Here's how the part is built. I have some questions about the finished solid (model axes, mm). A direction names the side the tool comes from. Coordinates: 2 decimals unless noted, no trailing zeros. Write each loop counter-clockwise with the first axis right and the second up, starting at its lowest first coordinate (ties: lowest second). Pieces come first, ordered by that corner, then holes.
(1) Thinking about a two-plate mould opening in X: for faces 1 (the cylindrical face through (4.77, 1.23, 1.5)), 2 (the flat face through (6, 0.5, -0.5)), 3 (the cylindrical face through (6.677, 1.972, -2.103)), which applies, released by +X, released by -X, zero draft, split by the parting line, or undercut?
(2) Imagine slicing it at B-B, the plane x = 0. List the corners of the cut face in (y, z) for me.
(3) Please list where these lines run through material, in increasing order: probe 1 along Z at (x, y) = (0, 0.9); probe 2 along Y at (x, z) = (-1, 5); probe 3 along X at (y, z) = (1.4, 3).
(4) Which directions (+Z, -Z, +X, -X, +Y, -Y) give clear straight access to the entire face, cutting with the end or side of a thin tool? Please do faces 4 (the flat face through (-6, 0.5, 0.5)), 5 (the flat face through (2, 2.5, -5)), 6 (the flat face through (-3, 4, -6)).
(5) Imagine slicing it at C-C, the plane y = 2. List the corners of the cut face in (x, z) for me.
(6) For pin 1 Ø8 at (x, z) = (0, 0) entering from -Y; pin 2 Ø0.8 at (x, z) = (-6, 0) entering from -Y; pin 3 Ø1.1 at (x, y) = (-6, 0.5) entering from +Z; pin 4 Ø1.5 at (y, z) = (1.5, -1.5) entering from +X, each with a flat end and sliding along its axis, tell me the tip position at first contact or that it passes through.
(7) Imagine slicing it at D-D, the plane x = 6. List the corners of the cut face in (y, z) for me.
(8) Imagine slicing it at A-A, the plane z = 0. List the corners of the cut face in (x, y) for me.
```python
from build123d import *

# Parameters (mm, degrees)
SKETCH1_R           = 7
BOSS_EXTRUDE1_DEPTH = 4
SKETCH2_R           = 6.25
CUT_EXTRUDE1_DEPTH  = 1.5
SKETCH3_R           = 5
CUT_EXTRUDE2_DEPTH  = 5
SKETCH4_W           = 16
SKETCH4_H           = 1
CUT_EXTRUDE3_DEPTH  = 1


with BuildPart() as part:
    # Sketch1 → Boss-Extrude1 (new body)
    with BuildSketch(Plane(origin=(0, 0, 0), x_dir=(1, 0, 0), z_dir=(0, 1, 0))):
        Circle(SKETCH1_R)
    extrude(amount=BOSS_EXTRUDE1_DEPTH)

    # Sketch2 → Cut-Extrude1 (cut)
    with BuildSketch(Plane(origin=(0, 4, 0), x_dir=(1, 0, 0), z_dir=(0, 1, 0))):
        Circle(SKETCH2_R)
    extrude(amount=-CUT_EXTRUDE1_DEPTH, mode=Mode.SUBTRACT)

    # Sketch3 → Cut-Extrude2 (cut, through all)
    with BuildSketch(Plane.XZ):
        Circle(SKETCH3_R)
    extrude(amount=-CUT_EXTRUDE2_DEPTH, mode=Mode.SUBTRACT)

    # Sketch4 → Cut-Extrude3 (cut)
    with BuildSketch(Plane.XZ):
        Rectangle(SKETCH4_W, SKETCH4_H)
    extrude(amount=-CUT_EXTRUDE3_DEPTH, mode=Mode.SUBTRACT)


solid = part.part
```
Recorded:
1. face 1: undercut
1. face 2: zero draft
1. face 3: split by the parting line
2. outline: (0, -7) - (4, -7) - (4, -6.25) - (2.5, -6.25) - (2.5, -5) - (0, -5) - close; (0, 5) - (2.5, 5) - (2.5, 6.25) - (4, 6.25) - (4, 7) - (0, 7) - close
3. probe 1: z = -7 to -5, 5 to 7
3. probe 2: y = 0 to 2.5
3. probe 3: x = -6.32 to -4, 4 to 6.32
4. face 4: +X, -X, -Y
4. face 5: +Y
4. face 6: +Z, -Z, +X, -X, +Y
5. outline: circle Ø14 at (0, 0); hole circle Ø10 at (0, 0)
6. pin 1: passes through
6. pin 2: stops at y = 1
6. pin 3: stops at z = 4.39
6. pin 4: stops at x = 6.96
7. outline: (0, -3.61) - (4, -3.61) - (4, -1.75) - (2.5, -1.75) - (2.5, 1.75) - (4, 1.75) - (4, 3.61) - (0, 3.61) - (0, 0.5) - (1, 0.5) - (1, -0.5) - (0, -0.5) - close
8. outline: (-7, 1) - (-5, 1) - (-5, 2.5) - (-6.25, 2.5) - (-6.25, 4) - (-7, 4) - close; (5, 1) - (7, 1) - (7, 4) - (6.25, 4) - (6.25, 2.5) - (5, 2.5) - close
